from build123d import *

# Parameters (mm, degrees)
FILLET1_R                = 3
BOSS_EXTRUDE4_REACH      = 44.135
BOSS_EXTRUDE4_END_RADIUS = 15.45
SKETCH3_W                = 7
SKETCH3_H                = 1.5
BOSS_EXTRUDE5_START      = -5
SKETCH4_R                = 1.75
BOSS_EXTRUDE5_DEPTH      = 5
CUT_EXTRUDE1_DEPTH       = 3.92
CUT_EXTRUDE1_DEPTH_BACK  = 3.19


with BuildPart() as part:
    # Sketch2 → Revolve1 (revolve)
    with BuildSketch(Plane.XY, mode=Mode.PRIVATE) as revolve1_sk:
        Polygon((3.5, 6), (15.45, 6), (15.45, 0), (16.65, 0), (16.65, -1.5), (17.95, -1.5), (17.95, 0), (17.95, 7.6), (5, 7.6), (5, 16), (3.5, 16), align=None)
    revolve(revolve1_sk.sketch.rotate(Axis((0, 0, 0), (0, 1, 0)), 90), axis=Axis((0, 0, 0), (0, 1, 0)))

    # Fillet1
    fillet1_edges = [part.edges().sort_by_distance(p)[0] for p in [
        (0, 7.6, 5),
    ]]
    fillet(fillet1_edges, radius=FILLET1_R)

    # Boss-Extrude4: up to this cylinder (the profile starts outside it)
    boss_extrude4_end = Plane(origin=(0, -0.75, 0), z_dir=(0, -1, 0)) * Cylinder(BOSS_EXTRUDE4_END_RADIUS, 120.17, mode=Mode.PRIVATE)
    # Sketch3 → Boss-Extrude4 (add, up to the surface)
    with BuildSketch(Plane(origin=(0, 0, 16.65), x_dir=(-1, 0, 0), z_dir=(0, 0, -1)), mode=Mode.PRIVATE) as boss_extrude4_sk1:
        with Locations((0, -0.75)):
            Rectangle(SKETCH3_W, SKETCH3_H)
    boss_extrude4_tool1 = extrude(boss_extrude4_sk1.sketch, amount=BOSS_EXTRUDE4_REACH, mode=Mode.PRIVATE) - boss_extrude4_end
    add(boss_extrude4_tool1.solids().sort_by_distance((0, -0.75, 16.65))[0])

    # Sketch4 → Boss-Extrude5 (add)
    with BuildSketch(Plane.XZ.offset(1.5).offset(BOSS_EXTRUDE5_START)):
        with BuildLine():
            Line((-21, -4), (-17.498642805, -4))
            ThreePointArc((-17.498642805, -4), (-17.95, 0), (-17.498642805, 4))
            Line((-17.498642805, 4), (-21, 4))
            ThreePointArc((-21, 4), (-25, 0), (-21, -4))
        make_face()
        with Locations(Location((-21, 0, 0), (0, 0, 270))):
            Circle(SKETCH4_R, mode=Mode.SUBTRACT)
    boss_extrude5 = extrude(amount=BOSS_EXTRUDE5_DEPTH)

    # Mirror1: Boss-Extrude5 across plane
    add(boss_extrude5.mirror(Plane(origin=(0, 0, 0), x_dir=(0, 0, 1), z_dir=(1, 0, 0))))

    # Sketch5 → Cut-Extrude1 (cut, two sides: drawn at the far end of the back side and taken through both)
    with BuildSketch(Plane(origin=(0, 0, 16.65), x_dir=(-1, 0, 0), z_dir=(0, 0, -1)).offset(-CUT_EXTRUDE1_DEPTH_BACK)):
        with BuildLine():
            Line((2.5, -1.5), (-2.5, -1.5))
            ThreePointArc((-2.5, -1.5), (0, -0.830127019), (2.5, -1.5))
        make_face()
    extrude(amount=CUT_EXTRUDE1_DEPTH + CUT_EXTRUDE1_DEPTH_BACK, mode=Mode.SUBTRACT)


solid = part.part
Read the model definition and answer for the solid it produces. Units are mm, in the model's axes. A direction names the side the tool comes from. Give positions to 0.01 mm unless a question says otherwise; leave off trailing zeros. Loops run counter-clockwise (first coordinate to the right, second up) from the corner with the lowest first, then second, coordinate; pieces in that order, holes last. Notation, with made-up numbers: (-18.5, 67) -> (39.5, 67) arc R25 cw to (39.5, 93) -> close; hole circle Ø9 at (65, 4.5). An arc over 180 degrees is marked (long way). Answer as CSV lines item,"result".
Item 1: Consider line 1 (X direction, y = -0.9, z = 0); line 2 (X direction, y = 0.8, z = 0); line 3 (Z direction, x = 21, y = 1.9). Determine where each line is inside the solid, lowest interval first. Write a range as [from, to].
Returned:
line 1,"x = [-25, -22.75], [-19.25, -16.65], [16.65, 19.25], [22.75, 25]"
line 2,"x = [-25, -22.75], [-19.25, -15.45], [15.45, 19.25], [22.75, 25]"
line 3,"z = [-4, -1.75], [1.75, 4]"
Item 2: Find section A-A on x = 0. Give the vertices of the cut face in (y, z).
Returned:
outline,"(-1.5, -17.95) -> (7.6, -17.95) -> (7.6, -8) arc R3 cw to (10.6, -5) -> (16, -5) -> (16, -3.5) -> (6, -3.5) -> (6, -15.45) -> (0, -15.45) -> (0, -16.65) -> (-1.5, -16.65) -> close; (-0.83, 15.45) -> (6, 15.45) -> (6, 3.5) -> (16, 3.5) -> (16, 5) -> (10.6, 5) arc R3 cw to (7.6, 8) -> (7.6, 17.95) -> (-0.83, 17.95) -> close"
Item 3: Find section C-C on y = 2.5. Give the vertices of the cut face in (x, z).
Returned:
outline,"(-21, -4) -> (-17.5, -4) arc R17.95 ccw to (17.5, -4) -> (21, -4) arc R4 ccw to (21, 4) -> (17.5, 4) arc R17.95 ccw to (-17.5, 4) -> (-21, 4) arc R4 ccw to start; hole circle Ø3.5 at (-21, 0); hole circle Ø30.9 at (0, 0); hole circle Ø3.5 at (21, 0)"
Item 4: Find section B-B on z = 0. State how many separate pieces and enclosed holes the cut face has, plus the area to 3 significant figures.
Returned:
separate pieces,"4"
enclosed holes,"0"
area,"145 mm²"
Item 5: Each of these flat-tipped pins is pushed along its axis until it touches: pin 1 (1.4 mm diameter, centred on y = -1, z = 15.5, fed in from +X); pin 2 (2 mm diameter, centred on y = 13, z = 1, fed in from +X); pin 3 (18.5 mm diameter, centred on x = 0, z = 0, fed in from -Y); pin 4 (6.5 mm diameter, centred on x = 0, z = 0, fed in from +Y). Where does it stop, or does it pass through?
Returned:
pin 1,"stops at x = 10.16"
pin 2,"stops at x = 5"
pin 3,"stops at y = 6"
pin 4,"passes through"
Item 6: Find section D-D on x = -10.5. Give the vertices of the cut face in (y, z).
Returned:
outline,"(-1.5, -14.56) -> (7.6, -14.56) -> (7.6, 14.56) -> (-1.5, 14.56) -> (-1.5, 12.92) -> (0, 12.92) -> (0, 11.33) -> (6, 11.33) -> (6, -11.33) -> (0, -11.33) -> (0, -12.92) -> (-1.5, -12.92) -> close"
Item 7: For faces 1 (the face through (-19, 1, -4)), 2 (the face through (0, 13, 5)), 3 (the face through (0.04, -0.83, 16.62)), 4 (the face through (-4, 6, 0)), determine the directions among +Z, -Z, +X, -X, +Y, -Y from which every point of the face is accessible in a straight line to the end or side of a thin tool.
Returned:
face 1,"-Z, -X, +Y, -Y"
face 2,"+Y"
face 3,"+Z, -Y"
face 4,"-Y"
